```python
from build123d import *

# Parameters (mm, degrees)
BOSS_EXTRU_1_DEPTH           = 16
ENL_V_MAT_EXTRU_1_DEPTH      = 203.869416128
ENL_V_MAT_EXTRU_1_DEPTH_BACK = 203.869416128
ESQUISSE2_R                  = 3


with BuildPart() as part:
    # Esquisse1 → Boss.-Extru.1 (new body)
    with BuildSketch(Plane.XY):
        Polygon((0, 0), (200, 0), (200, 30), (150, 30), (0, 15), align=None)
    extrude(amount=BOSS_EXTRU_1_DEPTH)

    # Esquisse2 → Enlèv. mat.-Extru.1 (cut, two sides: drawn at the far end of the back side and taken through both)
    with BuildSketch(Plane.XZ.offset(-ENL_V_MAT_EXTRU_1_DEPTH_BACK)):
        with Locations(Location((10, 8, 0), (0, 0, 180))):
            Circle(ESQUISSE2_R)
    extrude(amount=ENL_V_MAT_EXTRU_1_DEPTH + ENL_V_MAT_EXTRU_1_DEPTH_BACK, mode=Mode.SUBTRACT)


solid = part.part
```
Verification items for the finished model (mm, model axes). Coordinates: 2 decimals unless noted, no trailing zeros. Loops run counter-clockwise (first coordinate to the right, second up) from the corner with the lowest first, then second, coordinate; pieces in that order, holes last. Notation, with made-up numbers: (70, 57) - (122, 57) arc R13 ccw to (122, 70) - close; hole circle Ø5 at (88.25, 87). An arc over 180 degrees is marked (long way). Answer as a JSON object with one key per item and string values.
(1) Cross-section at B-B, the plane z = 8. Record the boundary of the cut face in (x, y).
Response:
{"outline": "(0, 0) - (7, 0) - (7, 15.7) - (0, 15) - close; (13, 0) - (200, 0) - (200, 30) - (150, 30) - (13, 16.3) - close"}
(2) Cross-section at C-C, the plane y = 19.5. Record the boundary of the cut face in (x, z).
Response:
{"outline": "(45, 0) - (200, 0) - (200, 16) - (45, 16) - close"}
(3) Cross-section at A-A, the plane x = 10. Record the boundary of the cut face in (y, z), then the cut area to 3 significant figures.
Response:
{"outline": "(0, 0) - (16, 0) - (16, 5) - (0, 5) - close; (0, 11) - (16, 11) - (16, 16) - (0, 16) - close", "area": "160 mm²"}
(4) Scan lines: line 1 along X through (y, z) = (5.75, 8); line 2 along Z through (x, y) = (10, 9.5); line 3 along X through (y, z) = (12.5, 7). Record each from-to range of solid material in increasing order.
Response:
{"line 1": "x = 0 to 7, 13 to 200", "line 2": "z = 0 to 5, 11 to 16", "line 3": "x = 0 to 7.17, 12.83 to 200"}
(5) Mould release check, pull along Z, two halves, no side actions. Record for faces 1 (the flat face through (121, 12, 16)), 2 (the flat face through (200, 15, 8)), 3 (the cylindrical face through (12.21, 8.28, 5.97)): pulls with the +Z half, pulls with the -Z half, needs draft (parallel to the pull), parting line crosses it, or undercut.
Response:
{"face 1": "pulls with the +Z half", "face 2": "needs draft", "face 3": "undercut"}
(6) Go/stop test with flat-tipped pins: pin 1 Ø8 at (x, z) = (10, 8) entering from +Y; pin 2 Ø5 at (x, z) = (63, 6) entering from +Y. Record where each tip stops, or that it passes through.
Response:
{"pin 1": "stops at y = 16.4", "pin 2": "stops at y = 21.55"}
